from build123d import *

# Parameters (mm, degrees)
F2_T = -5.08
F3_R = 2.53999
F4_R = 2.54
F5_R = 15.24


# Not quite as in the source:
# - a fillet or chamfer is up to 0.001 mm smaller than in the source, because OpenCascade refuses the exact size


with BuildPart() as f1:
    # F0 (on Front) → F1 (revolve)
    with BuildSketch(Plane.XZ):
        Polygon((-31.75, 3.175), (0, 3.175), (0, 180.975), (-76.2, 180.975), (-44.45, 0), (-38.1, 0), align=None)
    revolve(axis=Axis((0, 0, 92.075), (0, 0, -1)))

    # F2
    f2_openings = [f1.faces().sort_by_distance(p)[0] for p in [
        (0, 0, 180.975),
    ]]
    offset(amount=F2_T, openings=f2_openings, kind=Kind.INTERSECTION)

    # F3 (radius 2.54 in the source; OpenCascade refuses exactly that, so slightly less here)
    f3_edges = [f1.edges().sort_by_distance(p)[0] for p in [
        (76.2, 0, 180.975),
        (71.042415, 0, 180.975),
    ]]
    fillet(f3_edges, radius=F3_R)

    # F4
    f4_edges = [f1.edges().sort_by_distance(p)[0] for p in [
        (44.45, 0, 0),
        (38.1, 0, 0),
    ]]
    fillet(f4_edges, radius=F4_R)

    # F5
    f5_edges = [f1.edges().sort_by_distance(p)[0] for p in [
        (31.75, 0, 3.175),
    ]]
    fillet(f5_edges, radius=F5_R)


solid = f1.part
Here's how the part is built. I have some questions about the finished solid (model axes, mm). A direction names the side the tool comes from. Round coordinates to 2 decimals unless told otherwise and drop trailing zeros. Loops run counter-clockwise (first coordinate to the right, second up) from the corner with the lowest first, then second, coordinate; pieces in that order, holes last.
1. Which directions (+Z, -Z, +X, -X, +Y, -Y) give clear straight access to the entire face, cutting with the end or side of a thin tool? Please do faces 4 (the face through (0, 0, 8.255)), 5 (the face through (0, 0, 3.175)).
Answer list:
face 4: +Z
face 5: -Z
2. For P1, Ø12, axis at x = -14.5, y = -5.5, coming from the +Z side (3 decimals); P2, Ø8, axis at y = 7, z = 75.5, coming from the +X side; P3, Ø2, axis at y = 21.5, z = 92, coming from the +X side, each with a flat end and sliding along its axis, tell me the tip position at first contact or that it passes through.
Answer list:
P1: stops at z = 8.255
P2: stops at x = 58.09
P3: stops at x = 57.06
3. We'd pull the mould along Y, two halves only. Please class faces 1 (the face through (44.92, -34.44, 69.27)), 2 (the face through (4.6, 34.8, 1.5)), 3 (the face through (-19, -34, 0)): +Y half, -Y half, draft (parallel to the pull), parting line (faces both ways), or undercut.
Answer list:
face 1: parting line
face 2: undercut
face 3: draft
4. If we section it at C-C on z = 63: Write out the boundary of the cut face in (x, y), plus the area to 3 significant figures.
Answer list:
outline: circle Ø111.01 at (0, 0); hole circle Ø100.69 at (0, 0)
area: 1,720 mm2
5. If I drill on line 1 along Y through (x, z) = (-13, 68); line 2 along X through (y, z) = (-7, 144.5); line 3 along Y through (x, z) = (-28, 23), over which ranges is the centre line in solid material (lowest first)?
Answer list:
line 1: y = -54.86 to -49.55, 49.55 to 54.86
line 2: x = -69.45 to -64.26, 64.26 to 69.45
line 3: y = -39.58 to -33.06, 33.06 to 39.58
